Part model, mm, in its own coordinate system. A direction names the side the tool comes from. Coordinates: 2 decimals unless noted, no trailing zeros. Order: outer loops, then holes, each group sorted by start corner. A loop starts at its lowest first (then second) coordinate and runs counter-clockwise, first axis right, second up. Notation, with made-up numbers: (68.25, -18) - (95.25, -18) arc R31 ccw to (95.25, 15) - close; hole circle Ø11 at (4.5, 3.25). An arc over 180 degrees is marked (long way). Use a Markdown table: item, result. Add a question column.
1) Wall check: L1, parallel to X at y = 3.9, z = 0; L2, parallel to X at y = 22, z = -14.05; L3, parallel to Y at x = -42, z = -9.25. Give the ranges that are in metal, low to high. Write a range as [from, to].
2) Tool access for faces 4 (the face through (-27, 5, 5)), 5 (the face through (-24.795, 22.211, -11.183)), 6 (the face through (0, 20, -7)), 7 (the face through (-7, 20, -10)): list every direction of +Z, -Z, +X, -X, +Y, -Y with a clear straight run to the whole face (end or side of a thin tool).
3) Saw through at D-D on z = 11.75. List the corners of the cut face in (x, y), then the cut area to 3 significant figures.
4) Saw through at B-B on x = -30. List the corners of the cut face in (y, z).
5) Drop flat-ended pins along their axis: P1, Ø5, axis at x = -18, y = 20, coming from the +Z side; P2, Ø12.5, axis at x = -37.5, z = 6.5, coming from the +Y side; P3, Ø8, axis at x = -1.5, y = 27, coming from the +Z side; P4, Ø8.5, axis at x = -20, y = 22, coming from the -Z side. Give the stop position or say it passes through.
6) Saw through at A-A on z = 0. List the corners of the cut face in (x, y).
7) Saw through at C-C on y = 37. List the corners of the cut face in (x, z).
8) Two-plate mould, pull along Y, no slides. Class faces 1 (the face through (18.38, 26.76, -11.18)), 2 (the face through (-10.986, 30.01, 3.103)), 3 (the face through (-12, 3, 15)): +Y half, -Y half, draft (parallel to the pull), parting line (faces both ways), or undercut.
```python
from build123d import *

# Parameters (mm, degrees)
SKETCH1_W                     = 30
SKETCH1_H                     = 30
BOSS_EXTRUDE1_DEPTH           = 30
SKETCH2_W                     = 20
SKETCH2_H                     = 20
CUT_EXTRUDE1_DEPTH            = 37.742346142
SKETCH3_W                     = 30
SKETCH3_H                     = 5
BOSS_EXTRUDE2_DEPTH           = 40
SKETCH4_R                     = 5.5
SKETCH4_R_2                   = 1.8
CUT_EXTRUDE2_DEPTH            = 65.420493634
CUT_EXTRUDE3_DEPTH            = 63.24949799
SKETCH5_W                     = 5
SKETCH5_H                     = 25
BOSS_EXTRUDE4_DEPTH           = 34
CHAMFER1_SIZE                 = 25
SKETCH8_R                     = 2.1
CUT_EXTRUDE4_DEPTH            = 63.657800791
SKETCH9_W                     = 5
SKETCH9_H                     = 30
BOSS_EXTRUDE5_DEPTH           = 12
CHAMFER2_SIZE                 = 10
CHAMFER2_SIZE2                = 5.773502692
SKETCH10_R                    = 2.1
CUT_EXTRUDE5_DEPTH            = 63.657800791
BODY_MOVE_COPY1_START         = -15
BODY_MOVE_COPY1_DEPTH         = 31
BODY_MOVE_COPY1_START_2       = -10
BODY_MOVE_COPY1_2_DEPTH       = 26
BODY_MOVE_COPY1_3_OUTLINE_W   = 34
BODY_MOVE_COPY1_3_OUTLINE_H   = 5
BODY_MOVE_COPY1_3_DEPTH       = 30
BODY_MOVE_COPY1_4_DEPTH       = 5
BODY_MOVE_COPY1_5_OUTLINE_R   = 5.5
BODY_MOVE_COPY1_5_OUTLINE_R_2 = 1.8
BODY_MOVE_COPY1_5_DEPTH       = 5
SKETCH11_W                    = 3
SKETCH11_H                    = 25
CUT_EXTRUDE6_DEPTH            = 25
SKETCH12_W                    = 25
SKETCH12_H                    = 25
CUT_EXTRUDE7_DEPTH            = 60.380131357
SKETCH13_W                    = 3
SKETCH13_H                    = 6
SKETCH13_W_2                  = 6
SKETCH13_H_2                  = 3
BOSS_EXTRUDE6_DEPTH           = 30
SKETCH14_R                    = 4.8
CUT_EXTRUDE9_DEPTH            = 2.4
CHAMFER3_SIZE                 = 12
CHAMFER3_SIZE2                = 25
FILLET1_R                     = 4
BOSS_EXTRUDE7_DEPTH           = 10
BOSS_EXTRUDE8_DEPTH           = 5
FILLET3_R                     = 4
FILLET4_R                     = 4


with BuildPart() as part:
    # Sketch1 → Boss-Extrude1 (new body)
    with BuildSketch(Plane(origin=(0, 0, 0), x_dir=(1, 0, 0), z_dir=(0, 1, 0))):
        Rectangle(SKETCH1_W, SKETCH1_H)
    extrude(amount=BOSS_EXTRUDE1_DEPTH)

    # Sketch2 → Cut-Extrude1 (cut, through all)
    with BuildSketch(Plane(origin=(0, 30, 0), x_dir=(1, 0, 0), z_dir=(0, 1, 0))):
        Rectangle(SKETCH2_W, SKETCH2_H)
    extrude(amount=-CUT_EXTRUDE1_DEPTH, mode=Mode.SUBTRACT)

    # Sketch3 → Boss-Extrude2 (add)
    with BuildSketch(Plane(origin=(15, 0, 0), x_dir=(0, 0, -1), z_dir=(1, 0, 0))):
        with Locations((0, 2.5)):
            Rectangle(SKETCH3_W, SKETCH3_H)
    extrude(amount=BOSS_EXTRUDE2_DEPTH)

    # Sketch4 → Cut-Extrude2 (cut, through all)
    with BuildSketch(Plane.XZ):
        with Locations(Location((31, 0, 0), (0, 0, 270))):
            Circle(SKETCH4_R)
        with Locations(Location((19, 0, 0), (0, 0, 270))):
            Circle(SKETCH4_R_2)
        with Locations(Location((43, 0, 0), (0, 0, 270))):
            Circle(SKETCH4_R_2)
    extrude(amount=-CUT_EXTRUDE2_DEPTH, mode=Mode.SUBTRACT)

    # Sketch7 → Cut-Extrude3 (cut, through all)
    with BuildSketch(Plane(origin=(0, 5, 0), x_dir=(1, 0, 0), z_dir=(0, 1, 0))):
        Polygon((15, -15), (49, -6), (49, 15), (55, 15), (55, -15), align=None)
    extrude(amount=-CUT_EXTRUDE3_DEPTH, mode=Mode.SUBTRACT)

    # Sketch5 → Boss-Extrude4 (add)
    with BuildSketch(Plane(origin=(15, 0, 0), x_dir=(0, 0, -1), z_dir=(1, 0, 0))):
        with Locations((12.5, 17.5)):
            Rectangle(SKETCH5_W, SKETCH5_H)
    extrude(amount=BOSS_EXTRUDE4_DEPTH)

    # Chamfer1
    chamfer1_edges = [part.edges().sort_by_distance(p)[0] for p in [
        (49, 30, -12.5),
    ]]
    chamfer(chamfer1_edges, length=CHAMFER1_SIZE)

    # Sketch8 → Cut-Extrude4 (cut, through all)
    with BuildSketch(Plane.XY.offset(-10)):
        with Locations((20, 22)):
            Circle(SKETCH8_R)
    extrude(amount=-CUT_EXTRUDE4_DEPTH, mode=Mode.SUBTRACT)

    # Sketch9 → Boss-Extrude5 (add)
    with BuildSketch(Plane.ZY.offset(15)):
        with Locations((-12.5, 15)):
            Rectangle(SKETCH9_W, SKETCH9_H)
    extrude(amount=BOSS_EXTRUDE5_DEPTH)

    # Chamfer2
    chamfer2_edges = [part.edges().sort_by_distance(p)[0] for p in [
        (-27, 30, -12.5),
        (-27, 0, -12.5),
    ]]
    chamfer2_side = [part.faces().sort_by_distance(p)[0] for p in [
        (-27, 15, -12.5),
    ]]
    chamfer(chamfer2_edges, length=CHAMFER2_SIZE, length2=CHAMFER2_SIZE2, reference=chamfer2_side[0])

    # Sketch10 → Cut-Extrude5 (cut, through all)
    with BuildSketch(Plane.XY.offset(-10)):
        with Locations((-19, 22)):
            Circle(SKETCH10_R)
    extrude(amount=-CUT_EXTRUDE5_DEPTH, mode=Mode.SUBTRACT)

    # Body-Move/Copy1: read off the stored shape, not the designer's step
    # Body-Move/Copy1 outline → Body-Move/Copy1 (cut)
    with BuildSketch(Plane.XY.offset(BODY_MOVE_COPY1_START)):
        Polygon((24, 30), (21.226497308, 30), (27, 20), (27, 10), (21.226497308, 0), (49, 0), (49, 5), align=None)
        with BuildLine():
            ThreePointArc((-19.5, 19.960392195), (-21.1, 22), (-19.5, 24.039607805))
            ThreePointArc((-19.5, 24.039607805), (-22.1, 22), (-19.5, 19.960392195))
        make_face()
        with BuildLine():
            ThreePointArc((19.5, 19.960392195), (17.9, 22), (19.5, 24.039607805))
            ThreePointArc((19.5, 24.039607805), (16.9, 22), (19.5, 19.960392195))
        make_face()
    extrude(amount=BODY_MOVE_COPY1_DEPTH, mode=Mode.SUBTRACT)

    # Body-Move_Copy1 2 outline → Body-Move_Copy1 2 (cut)
    with BuildSketch(Plane.XY.offset(BODY_MOVE_COPY1_START_2)):
        Polygon((24.113248654, 5), (15, 5), (15, 0), (21.226497308, 0), align=None)
    extrude(amount=BODY_MOVE_COPY1_2_DEPTH, mode=Mode.SUBTRACT)

    # Body-Move_Copy1 3 outline → Body-Move_Copy1 3 (add)
    with BuildSketch(Plane.XY.offset(BODY_MOVE_COPY1_START)):
        with Locations((-32, 2.5)):
            Rectangle(BODY_MOVE_COPY1_3_OUTLINE_W, BODY_MOVE_COPY1_3_OUTLINE_H)
    extrude(amount=BODY_MOVE_COPY1_3_DEPTH)

    # Body-Move_Copy1 4 outline → Body-Move_Copy1 4 (add)
    with BuildSketch(Plane.XY.offset(BODY_MOVE_COPY1_START)):
        Polygon((-27, 20), (-21.226497308, 30), (-24, 30), (-49, 5), (-24.113248654, 5), (-27, 10), align=None)
        with BuildLine():
            ThreePointArc((-19.5, 24.039607805), (-17.9, 22), (-19.5, 19.960392195))
            ThreePointArc((-19.5, 19.960392195), (-16.9, 22), (-19.5, 24.039607805))
        make_face()
        with BuildLine():
            ThreePointArc((19.5, 24.039607805), (21.1, 22), (19.5, 19.960392195))
            ThreePointArc((19.5, 19.960392195), (22.1, 22), (19.5, 24.039607805))
        make_face()
    extrude(amount=BODY_MOVE_COPY1_4_DEPTH)

    # Body-Move_Copy1 5 outline → Body-Move_Copy1 5 (cut)
    with BuildSketch(Plane(origin=(0, 0, 0), x_dir=(1, 0, 0), z_dir=(0, 1, 0))):
        with Locations((-31, 0)):
            Circle(BODY_MOVE_COPY1_5_OUTLINE_R)
        with Locations((-19, 0)):
            Circle(BODY_MOVE_COPY1_5_OUTLINE_R_2)
        with Locations((-43, 0)):
            Circle(BODY_MOVE_COPY1_5_OUTLINE_R_2)
        Polygon((-49, -15), (-15, -15), (-49, -6), align=None)
    extrude(amount=BODY_MOVE_COPY1_5_DEPTH, mode=Mode.SUBTRACT)

    # Sketch11 → Cut-Extrude6 (cut)
    with BuildSketch(Plane(origin=(0, 30, 0), x_dir=(1, 0, 0), z_dir=(0, 1, 0))):
        with Locations((-13.5, -2.5)):
            Rectangle(SKETCH11_W, SKETCH11_H)
    extrude(amount=-CUT_EXTRUDE6_DEPTH, mode=Mode.SUBTRACT)

    # Sketch12 → Cut-Extrude7 (cut, through all)
    with BuildSketch(Plane(origin=(0, 30, 0), x_dir=(1, 0, 0), z_dir=(0, 1, 0))):
        with Locations((2.5, -2.5)):
            Rectangle(SKETCH12_W, SKETCH12_H)
    extrude(amount=-CUT_EXTRUDE7_DEPTH, mode=Mode.SUBTRACT)

    # Sketch13 → Boss-Extrude6 (add)
    with BuildSketch(Plane(origin=(0, 30, 0), x_dir=(1, 0, 0), z_dir=(0, 1, 0))):
        with Locations((-8.5, 0)):
            Rectangle(SKETCH13_W, SKETCH13_H)
        with Locations((0, 8.5)):
            Rectangle(SKETCH13_W_2, SKETCH13_H_2)
    extrude(amount=-BOSS_EXTRUDE6_DEPTH)

    # Sketch14 → Cut-Extrude9 (cut)
    with BuildSketch(Plane.XY.offset(-10)):
        with Locations((-20, 22)):
            Circle(SKETCH14_R)
        with Locations((19, 22)):
            Circle(SKETCH14_R)
    extrude(amount=-CUT_EXTRUDE9_DEPTH, mode=Mode.SUBTRACT)

    # Chamfer3
    chamfer3_edges = [part.edges().sort_by_distance(p)[0] for p in [
        (-11, 30, 15),
    ]]
    chamfer3_side = [part.faces().sort_by_distance(p)[0] for p in [
        (-18, 30, -10.542718717),
    ]]
    chamfer(chamfer3_edges, length=CHAMFER3_SIZE, length2=CHAMFER3_SIZE2, reference=chamfer3_side[0])

    # Fillet1
    fillet1_edges = [part.edges().sort_by_distance(p)[0] for p in [
        (-49, 2.5, 6),
        (-15, 2.5, 15),
    ]]
    fillet(fillet1_edges, radius=FILLET1_R)

    # Sketch16 → Boss-Extrude7 (add)
    with BuildSketch(Plane(origin=(0, 30, 0), x_dir=(1, 0, 0), z_dir=(0, 1, 0))):
        Polygon((-12, -3), (-7, -3), (-7, 3), (-10, 3), (-10, 10), (-3, 10), (-3, 7), (3, 7), (3, 15), (-12, 15), align=None)
    extrude(amount=BOSS_EXTRUDE7_DEPTH)

    # Sketch17 → Boss-Extrude8 (add)
    with BuildSketch(Plane(origin=(0, 0, -15), x_dir=(-1, 0, 0), z_dir=(0, 0, -1))):
        Polygon((-21.226497308, 30), (-3, 40), (-3, 30), align=None)
        Polygon((12, 30), (12, 40), (24, 30), align=None)
    extrude(amount=-BOSS_EXTRUDE8_DEPTH)

    # Fillet3
    fillet3_edges = [part.edges().sort_by_distance(p)[0] for p in [
        (-11, 30, 3),
    ]]
    fillet(fillet3_edges, radius=FILLET3_R)

    # Fillet4
    # the kernel refuses this fillet: 4 mm, written as the material it takes off along each edge
    with BuildSketch(Plane(origin=(27, 10, -17.679491924), x_dir=(-0.500000000006737, -0.8660254037805489, 0), z_dir=(0, 0, 1))) as fillet4_piece_1:
        with BuildLine():
            CenterArc((FILLET4_R * 0.267949192435, -FILLET4_R), FILLET4_R, 90, 30)
            Line((-FILLET4_R * 0.232050807571, -FILLET4_R * 0.133974596219), (0, 0))
            Line((0, 0), (FILLET4_R * 0.267949192435, 0))
        make_face()
    extrude(amount=10.358983849, mode=Mode.SUBTRACT)
    with BuildSketch(Plane(origin=(27, 20, -17.679491924), x_dir=(-0.5000000000067392, 0.8660254037805477, 0), z_dir=(0, 0, 1))) as fillet4_piece_2:
        with BuildLine():
            CenterArc((FILLET4_R * 0.267949192435, FILLET4_R), FILLET4_R, 240, 30)
            Line((-FILLET4_R * 0.232050807571, FILLET4_R * 0.133974596219), (0, 0))
            Line((0, 0), (FILLET4_R * 0.267949192435, 0))
        make_face()
    extrude(amount=10.358983849, mode=Mode.SUBTRACT)
    with BuildSketch(Plane(origin=(21.226497308, 30, -17.796617535), x_dir=(0.5000000000067387, -0.8660254037805479, 0), z_dir=(0, 0, 1))) as fillet4_piece_3:
        with BuildLine():
            CenterArc((FILLET4_R * 0.27966175346, -FILLET4_R), FILLET4_R, 90, 31.248547441)
            Line((-FILLET4_R * 0.23908983086, -FILLET4_R * 0.145074977694), (0, 0))
            Line((0, 0), (FILLET4_R * 0.27966175346, 0))
        make_face()
    extrude(amount=10.59323507, mode=Mode.SUBTRACT)
    with BuildSketch(Plane(origin=(-24, 30, -15.453610172), x_dir=(0.7682212795973823, 0.6401843996644723, 0), z_dir=(0, 0, 1))) as fillet4_piece_4:
        with BuildLine():
            CenterArc((FILLET4_R * 0.0453610171873, -FILLET4_R), FILLET4_R, 90, 5.194428908)
            Line((-FILLET4_R * 0.0451747288553, -FILLET4_R * 0.0041067935323), (0, 0))
            Line((0, 0), (FILLET4_R * 0.0453610171873, 0))
        make_face()
    extrude(amount=5.907220344, mode=Mode.SUBTRACT)


solid = part.part
```
Results are:
| question | item | result |
|---|---|---|
| 1 | L1 | [-49, -44.8], [-41.2, -36.5], [-25.5, -20.8], [-17.2, -7] |
| 1 | L2 | [-32, -22.1], [-17.9, 16.9], [21.1, 25.85] |
| 1 | L3 | [0, 5] |
| 2 | face 4 | +Z, -X, +Y |
| 2 | face 5 | +Z |
| 2 | face 6 | +Z, +X, +Y, -Y |
| 2 | face 7 | +Y, -Y |
| 3 | outline | (-27.28, 0) - (-10, 0) - (-10, 11.77) - (-12, 11.77) - (-12, 5) - (-27.28, 5) - close |
| 3 | area | 99.9 mm2 |
| 4 | outline | (0, -15) - (24, -15) - (24, -10) - (5, -10) - (5, -5.41) - (0, -5.41) - close; (0, 5.41) - (5, 5.41) - (5, 11.03) - (0, 11.03) - close |
| 5 | P1 | z = -10 |
| 5 | P2 | y = 5 |
| 5 | P3 | z = -7 |
| 5 | P4 | z = -15 |
| 6 | outline | (-49, 0) - (-44.8, 0) - (-44.8, 5) - (-49, 5) - close; (-41.2, 0) - (-36.5, 0) - (-36.5, 5) - (-41.2, 5) - close; (-25.5, 0) - (-20.8, 0) - (-20.8, 5) - (-25.5, 5) - close; (-17.2, 0) - (-7, 0) - (-7, 40) - (-12, 40) - (-12, 5) - (-17.2, 5) - close |
| 7 | outline | (-15.6, -15) - (8.47, -15) - (8.47, -10) - (3, -10) - (3, -7) - (-3, -7) - (-3, -10) - (-10, -10) - (-10, -3) - (-7, -3) - (-7, 3) - (-12, 3) - (-12, -10) - (-15.6, -10) - close |
| 8 | face 1 | undercut |
| 8 | face 2 | +Y half |
| 8 | face 3 | draft |
